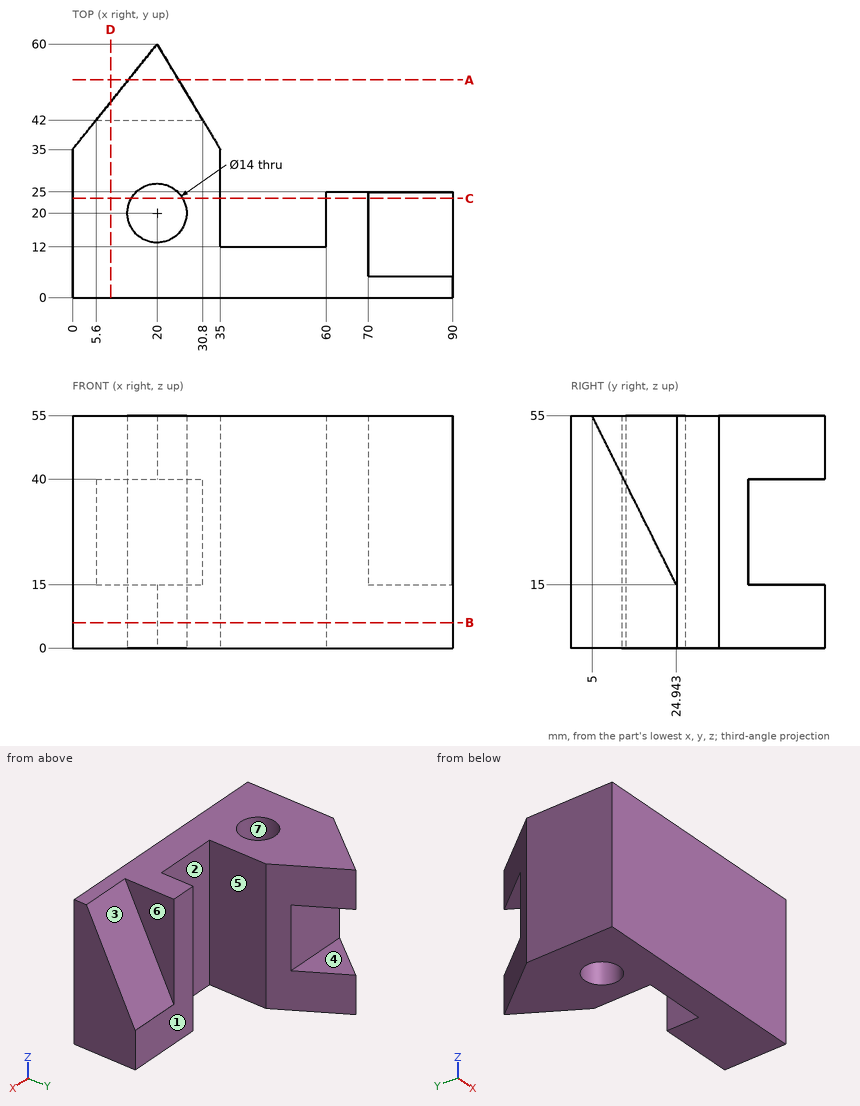
Study the drawing (mm; zero at the part's minimum x, y, z) and answer. A direction names the side the tool comes from. Coordinates: 2 decimals unless noted, no trailing zeros. Write each loop counter-clockwise with the first axis right and the second up, starting at its lowest first coordinate (ties: lowest second). Pieces come first, ordered by that corner, then holes. Notation, with made-up numbers: M 74.5,62.25 L 112.5,62.25 A25 cw 112.5,91.25 Z; hole C 73,74 d10. An arc over 180 degrees is marked long. Use a Markdown table: item, result. Add a question column.
1. Section D-D (x = 9) is taken. Give the vertices of the cut face in (y, z), plus the area to 3 significant figures.
2. Section B-B (z = 6) is taken. Give the vertices of the cut face in (x, y).
3. Section C-C (y = 23.5) is taken. Give the vertices of the cut face in (x, z).
4. Straight lines are drawn through the part: line 1 along Y through (x, z) = (61, 34.5); line 2 along Y through (x, z) = (42, 13); line 3 along Y through (x, z) = (20, 16). For each, find the intervals that lie inside material, in ascending order. Write a range as [from, to].
5. Section A-A (y = 51.5) is taken. Give the vertices of the cut face in (x, z), plus the area to 3 significant figures.
6. Which of the six approach directions +Z, -Z, +X, -X, +Y, -Y give full straight-line access (tool end or side, diameter ignored) to the marked faces 1, 2 and 3?
7. Given P1, Ø16, axis at y = 14.5, z = 43, coming from the +X side; P2, Ø8, axis at y = 33, z = 13, coming from the +X side; P3, Ø12.5, axis at x = 44, z = 26.5, coming from the +Y side, each flat-ended and moving along its own axis, determine where each tip first touches the part or whether it passes through.
8. For a pull along X with two mould halves and no side action, classify the marked faces 4, 5, 6 and 7 as +X half, -X half, draft (parallel to the pull), parting line (faces both ways), or undercut.
Data:
| question | item | result |
|---|---|---|
| 1 | outline | M 0,0 L 46.25,0 L 46.25,15 L 42,15 L 42,40 L 46.25,40 L 46.25,55 L 0,55 Z |
| 1 | area | 2,440 mm2 |
| 2 | outline | M 0,0 L 90,0 L 90,25 L 60,25 L 60,12 L 35,12 L 35,35 L 20,60 L 0,35 Z; hole C 20,20 d14 |
| 3 | outline | M 0,0 L 13.94,0 L 13.94,55 L 0,55 Z; M 26.06,0 L 35,0 L 35,55 L 26.06,55 Z; M 60,0 L 90,0 L 90,17.89 L 70,17.89 L 70,55 L 60,55 Z |
| 4 | line 1 | y = [0, 25] |
| 4 | line 2 | y = [0, 12] |
| 4 | line 3 | y = [0, 13], [27, 42] |
| 5 | outline | M 13.2,0 L 25.1,0 L 25.1,15 L 13.2,15 Z; M 13.2,40 L 25.1,40 L 25.1,55 L 13.2,55 Z |
| 5 | area | 357 mm2 |
| 6 | face 1 | +Z, -Z, +X, +Y |
| 6 | face 2 | +Z, -Z, +Y |
| 6 | face 3 | +Z, +X, +Y |
| 7 | P1 | stops at x = 90 |
| 7 | P2 | stops at x = 35 |
| 7 | P3 | stops at y = 12 |
| 8 | face 4 | draft |
| 8 | face 5 | undercut |
| 8 | face 6 | +X half |
| 8 | face 7 | undercut |
